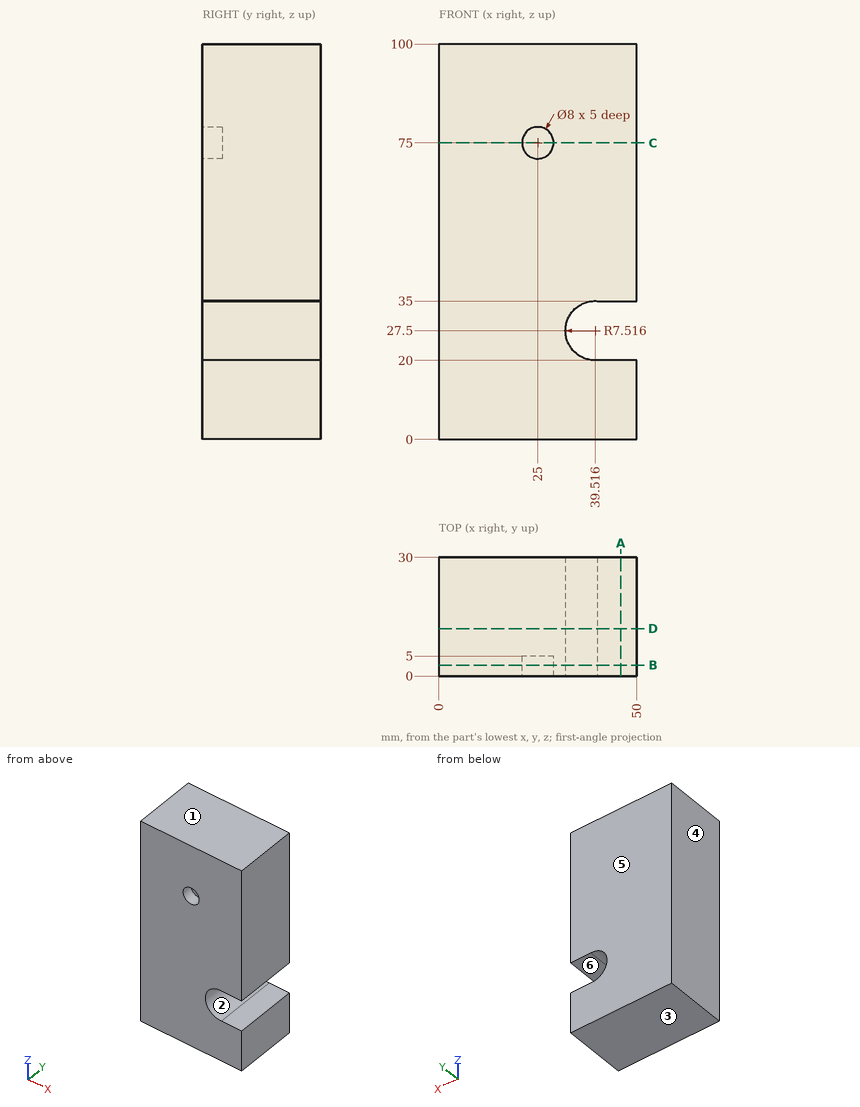
Could you check a few things on this drawing? It's one solid part, dimensions in mm from its lowest x, y, z. A direction names the side the tool comes from. Coordinates: 2 decimals unless noted, no trailing zeros. Write each loop counter-clockwise with the first axis right and the second up, starting at its lowest first coordinate (ties: lowest second). Pieces come first, ordered by that corner, then holes. Notation, with made-up numbers: (13.25, 49.25) - (28.25, 49.25) arc R14 cw to (28.25, 71.25) - close; hole circle Ø9 at (-3, -40). An arc over 180 degrees is marked (long way). Return JSON: item names as keys, results as strings. Group by question number.
Item 1: If we section it at B-B (y = 2.75): Write out the boundary of the cut face in (x, z) (1 decimal).
Item 2: We'd pull the mould along Z, two halves only. Please class the marked faces 1, 2, 3 and 4: pulls with the +Z half, pulls with the -Z half, needs draft (parallel to the pull), parting line crosses it, or undercut.
Item 3: If we section it at A-A (x = 46): Write out the boundary of the cut face in (y, z), then the cut area to 3 significant figures.
Item 4: If we section it at D-D (y = 12): Write out the boundary of the cut face in (x, z) (1 decimal), then the cut area to 3 significant figures.
Item 5: If we section it at C-C (z = 75): Write out the boundary of the cut face in (x, y).
Item 6: Which directions (+Z, -Z, +X, -X, +Y, -Y) give clear straight access to the entire face, cutting with the end or side of a thin tool? Please do the marked faces 5 and 6.
Item 7: Please list where these lines run through material, in increasing order: probe 1 along Z at (x, y) = (25, 3.5); probe 2 along Z at (x, y) = (42.5, 20.5); probe 3 along Y at (x, z) = (26, 75).
Return value:
{
 "1": {"outline": "(0, 0) - (50, 0) - (50, 20) - (40, 20) arc R7.5 cw (long way) to (40, 35) - (50, 35) - (50, 100) - (0, 100) - close; hole circle Ø8 at (25, 75)"},
 "2": {"face 1": "pulls with the +Z half", "face 2": "undercut", "face 3": "pulls with the -Z half", "face 4": "needs draft"},
 "3": {"outline": "(0, 0) - (30, 0) - (30, 20) - (0, 20) - close; (0, 35) - (30, 35) - (30, 100) - (0, 100) - close", "area": "2,550 mm^2"},
 "4": {"outline": "(0, 0) - (50, 0) - (50, 20) - (40, 20) arc R7.5 cw (long way) to (40, 35) - (50, 35) - (50, 100) - (0, 100) - close", "area": "4,750 mm^2"},
 "5": {"outline": "(0, 0) - (21, 0) - (21, 5) - (29, 5) - (29, 0) - (50, 0) - (50, 30) - (0, 30) - close"},
 "6": {"face 5": "+Z, -Z, +X, -X, +Y", "face 6": "+X, +Y, -Y"},
 "7": {"probe 1": "z = 0 to 71, 79 to 100", "probe 2": "z = 0 to 20, 35 to 100", "probe 3": "y = 5 to 30"}
}
